from build123d import *

# Parameters (mm, degrees)
SWEEP_1_PROFILE_R = 2.5
SKETCH_10_W       = 10
SKETCH_10_H       = 10
EXTRUDE_1_DEPTH   = 5
SKETCH_11_W       = 12.093454082
SKETCH_11_H       = 15.976124646
EXTRUDE_2_DEPTH   = 8


with BuildPart() as part:
    # 扫描1: sweep along a curve in space
    with BuildLine() as sweep_1_path:
        Line((0, 0, 0), (0, 0, -11.265055353))
        ThreePointArc((11.293060244, 0, -49.389787804), (2.882618559, 0, -31.146129482), (0, 0, -11.265055353))
        Line((11.293060244, 0, -49.389787804), (16.33917105, 0, -57.160117038))
        ThreePointArc((27.231951751, 20, -73.933528397), (24.04153015, 5.857864376, -69.020709954), (16.33917105, 0, -57.160117038))
        Line((27.231951751, 20, -73.933528397), (27.231951751, 44, -73.933528397))
    # 扫描1 profile (on start of the path) → 扫描1 (sweep)
    with BuildSketch(Plane(origin=(0, 0, 0), x_dir=(-1, 0, 0), z_dir=(0, 0, -1))):
        Circle(SWEEP_1_PROFILE_R)
    sweep(path=sweep_1_path.line)

    # 草图10 → 凸台-拉伸1 (add)
    with BuildSketch(Plane.XY):
        Rectangle(SKETCH_10_W, SKETCH_10_H)
    extrude(amount=EXTRUDE_1_DEPTH)

    # 草图11 → 凸台-拉伸2 (add)
    with BuildSketch(Plane(origin=(0, 44, 0), x_dir=(1, 0, 0), z_dir=(0, 1, 0))):
        with Locations((27.231951751, 70.082405306)):
            Rectangle(SKETCH_11_W, SKETCH_11_H)
    extrude(amount=EXTRUDE_2_DEPTH)


solid = part.part
Design review of the part built by this model. Coordinates are the model's own, in mm. A direction names the side the tool comes from. Coordinates: 2 decimals unless noted, no trailing zeros. Write each loop counter-clockwise with the first axis right and the second up, starting at its lowest first coordinate (ties: lowest second). Pieces come first, ordered by that corner, then holes. Notation, with made-up numbers: (-3, 30.25) -> (23, 30.25) arc R24 cw to (23, 46.25) -> close; hole circle Ø4 at (1, 85). An arc over 180 degrees is marked (long way). Write each question's results on one line, items separated by ' | '. Start each with the question number.
(1) For line 1 along Z through (x, y) = (27.5, 22); line 2 along Y through (x, z) = (16.5, -57.5); line 3 along Z through (x, y) = (28.5, 27), list the stretches that pass through material, from the lowest coordinate up. Write a range as from..to.
(2) Tool access review of faces 1 (the face through (21.185, 48, -70)), 2 (the face through (29.267, 32.168, -72.481)), 3 (the face through (0, -5, 2)): name each direction out of +Z, -Z, +X, -X, +Y, -Y from which nothing blocks a thin tool from reaching the whole face with its end or side.
(3) Clearance check with flat-ended pins moving along their axes: P1, Ø5, axis at x = 23, y = 6, coming from the -Z side; P2, Ø11, axis at x = 2.5, y = 0.5, coming from the -Z side; P3, Ø8, axis at x = 6, z = -49, coming from the +Y side; P4, Ø10, axis at y = 9, z = -54, coming from the -X side. State where each tip first meets the part, or that it passes through.
(4) The part is to be moulded in two halves that separate along Z. For faces 4 (the face through (-2, 2, 0)), 5 (the face through (0.54, -2.44, -5.71)), 6 (the face through (5, 0, 2)), 7 (the face through (27, 48, -62.094)), say which applies: pulls with the +Z half, pulls with the -Z half, needs draft (parallel to the pull), parting line crosses it, or undercut.
(5) Take a section at B-B on y = 21.5. Write out the cut boundary in (x, z).
(6) Take a section at A-A on z = -6. Write out the cut boundary in (x, y), and give its area (3 significant figures).
Results found:
1) line 1: z = -76.42..-71.45 | line 2: y = -2.5..2.5 | line 3: z = -76.09..-71.78
2) face 1: +Z, -Z, -X, +Y | face 2: none | face 3: +Z, -Z, +X, -X, -Y
3) P1: stops at z = -73.27 | P2: stops at z = -48.82 | P3: stops at y = 2.48 | P4: passes through
4) face 4: undercut | face 5: undercut | face 6: needs draft | face 7: pulls with the +Z half
5) outline: circle Ø5 at (27.23, -73.93)
6) outline: circle Ø5 at (0, 0) | area: 19.6 mm2
